from build123d import *

# Parameters (mm, degrees)
BOSS_EXTRUDE1_DEPTH = 26
SKETCH2_W           = 75
SKETCH2_H           = 20
CUT_EXTRUDE1_DEPTH  = 1
SKETCH4_W           = 75
SKETCH4_H           = 20
CUT_EXTRUDE2_DEPTH  = 1
SKETCH5_W           = 14.75
SKETCH5_H           = 20
CUT_EXTRUDE3_DEPTH  = 46.882459228
SKETCH6_R           = 3.375
SKETCH6_R_2         = 1.375
BOSS_EXTRUDE2_DEPTH = 5


with BuildPart() as part:
    # Sketch1 → Boss-Extrude1 (new body)
    with BuildSketch(Plane.XY):
        Polygon((27.035253752, 0), (-27.035253752, 0), (-37.5, 3.790622591), (-37.5, 6.790622591), (-27.035253752, 3), (27.035253752, 3), (37.5, 6.790622591), (37.5, 3.790622591), align=None)
    extrude(amount=BOSS_EXTRUDE1_DEPTH)

    # Sketch2 → Cut-Extrude1 (cut)
    with BuildSketch(Plane.XZ):
        with Locations((0, 13)):
            Rectangle(SKETCH2_W, SKETCH2_H)
    extrude(amount=-CUT_EXTRUDE1_DEPTH, mode=Mode.SUBTRACT)

    # Sketch4 → Cut-Extrude2 (cut)
    with BuildSketch(Plane.XZ.offset(-1)):
        with Locations((0, 13)):
            Rectangle(SKETCH4_W, SKETCH4_H)
    extrude(amount=-CUT_EXTRUDE2_DEPTH, mode=Mode.SUBTRACT)

    # Sketch5 → Cut-Extrude3 (cut, through all)
    with BuildSketch(Plane.XZ.offset(-2)):
        with Locations((0, 13)):
            Rectangle(SKETCH5_W, SKETCH5_H)
    extrude(amount=-CUT_EXTRUDE3_DEPTH, mode=Mode.SUBTRACT)

    # Sketch6 → Boss-Extrude2 (add)
    # profile 1 of 2: a face of its own
    with BuildSketch(Plane(origin=(0, 3, 0), x_dir=(1, 0, 0), z_dir=(0, 1, 0))):
        with Locations(Location((-17.205126876, -13, 0), (0, 0, 90))):
            Circle(SKETCH6_R)
        with Locations(Location((-17.205126876, -13, 0), (0, 0, 270))):
            Circle(SKETCH6_R_2, mode=Mode.SUBTRACT)
    # profile 2 of 2: a face of its own
    with BuildSketch(Plane(origin=(0, 3, 0), x_dir=(1, 0, 0), z_dir=(0, 1, 0))):
        with Locations(Location((17.205126876, -13, 0), (0, 0, 90))):
            Circle(SKETCH6_R)
        with Locations(Location((17.205126876, -13, 0), (0, 0, 90))):
            Circle(SKETCH6_R_2, mode=Mode.SUBTRACT)
    extrude(amount=BOSS_EXTRUDE2_DEPTH)


solid = part.part
Verification items for the finished model (mm, model axes). A direction names the side the tool comes from. Give positions to 0.01 mm unless a question says otherwise; leave off trailing zeros. Order: outer loops, then holes, each group sorted by start corner. A loop starts at its lowest first (then second) coordinate and runs counter-clockwise, first axis right, second up. Notation, with made-up numbers: M -3,17 L 8,17 A20 cw 8,34 Z; hole C 70.5,15.25 d7. An arc over 180 degrees is marked long. Answer as a JSON object with one key per item and string values. Group by question number.
1) Cross-section at D-D (x = 11). Enter the section's corners in (y, z).
2) Cross-section at A-A (x = -2.5). Enter the section's corners in (y, z), then the cut area to 3 significant figures.
3) Access from +Z, -Z, +X, -X, +Y, -Y to the whole of each face (thin tool, end or side, straight path). Record for faces 4 (the face through (-17.145, 5.465, 11.626)), 5 (the face through (-32.34, 4.92, 12.82)), 6 (the face through (-20, 2, 13)).
4) Cross-section at B-B (z = 5.75). Enter the section's corners in (x, y) (3 decimals), then the cut area to 3 significant figures.
5) Cross-section at C-C (z = 13). Enter the section's corners in (x, y) (3 decimals), then the cut area to 3 significant figures.
6) Scan lines: line 1 along Z through (x, y) = (5.5, 0.5); line 2 along Y through (x, z) = (-12.5, 3.75); line 3 along Z through (x, y) = (20, 7.75). Record each from-to range of solid material in increasing order. Write a range as [from, to].
7) Mould release check, pull along Z, two halves, no side actions. Record for faces 1 (the face through (1, 2, 26)), 2 (the face through (20, 2, 13)), 3 (the face through (-37.5, 5, 13)): released by +Z, released by -Z, zero draft, split by the parting line, or undercut.
8) Depth check by flat-ended pin: pin 1 Ø1 at (x, z) = (23, 17.5) entering from -Y; pin 2 Ø3 at (y, z) = (2.5, 18.5) entering from +X; pin 3 Ø12 at (x, z) = (27.5, 19.5) entering from +Y; pin 4 Ø3 at (x, z) = (30, 20.5) entering from +Y. Enter the tip coordinate at first touch or a pass-through.
Result sheet:
{
 "1": {"outline": "M 0,0 L 3,0 L 3,26 L 0,26 L 0,23 L 2,23 L 2,3 L 0,3 Z"},
 "2": {"outline": "M 0,0 L 3,0 L 3,3 L 0,3 Z; M 0,23 L 3,23 L 3,26 L 0,26 Z", "area": "18.0 mm2"},
 "3": {"face 4": "+Y", "face 5": "+Z, -Z, +Y", "face 6": "+X, -X, -Y"},
 "4": {"outline": "M -37.5,3.791 L -32.557,2 L -7.375,2 L -7.375,3 L -27.035,3 L -37.5,6.791 Z; M 7.375,2 L 32.557,2 L 37.5,3.791 L 37.5,6.791 L 27.035,3 L 7.375,3 Z", "area": "91.1 mm2"},
 "5": {"outline": "M -37.5,3.791 L -32.557,2 L -7.375,2 L -7.375,3 L -13.83,3 L -13.83,8 L -15.83,8 L -15.83,3 L -18.58,3 L -18.58,8 L -20.58,8 L -20.58,3 L -27.035,3 L -37.5,6.791 Z; M 7.375,2 L 32.557,2 L 37.5,3.791 L 37.5,6.791 L 27.035,3 L 20.58,3 L 20.58,8 L 18.58,8 L 18.58,3 L 15.83,3 L 15.83,8 L 13.83,8 L 13.83,3 L 7.375,3 Z", "area": "131 mm2"},
 "6": {"line 1": "z = [0, 3], [23, 26]", "line 2": "y = [2, 3]", "line 3": "z = [11.11, 14.89]"},
 "7": {"face 1": "released by +Z", "face 2": "undercut", "face 3": "zero draft"},
 "8": {"pin 1": "stops at y = 2", "pin 2": "stops at x = 37.5", "pin 3": "stops at y = 5.34", "pin 4": "stops at y = 4.62"}
}
